Input: part model. Units: mm. Frame: model coordinates. Face numbers are marked on the shaded views. Give positions to 0.01 mm unless a question says otherwise; leave off trailing zeros. Loops run counter-clockwise (first coordinate to the right, second up) from the corner with the lowest first, then second, coordinate; pieces in that order, holes last. Notation, with made-up numbers: (45.25, 61.5) - (63.25, 61.5) arc R19 ccw to (63.25, 86.5) - close; hole circle Ø3 at (88, -32.5). An arc over 180 degrees is marked (long way). Answer as a JSON object with one key per item and string values. Group by question number.
(1) Section query D-D (y = 1.1). Return loops of the section in (x, z), plus the area to 3 significant figures.
(2) Mould query, pull axis X, two halves, no side actions, for the marked faces 1 and 2. Classes: +X half, -X half, draft (parallel to the pull), parting line (faces both ways), or undercut.
(3) Section query B-B (z = -68). Return loops of the section in (x, y), plus the area to 4 significant figures.
(4) Material intervals for L1, parallel to Z at x = 40.8, y = 0.2; L2, parallel to X at y = 0.3, z = -68; L3, parallel to Z at x = 28, y = 1.85, sorted ascending.
(5) Pin query (flat end, axial travel): P1, Ø3.5, axis at x = 40.8, z = -68, coming from the +Y side; P2, Ø0.8, axis at x = 19, y = 1.5, coming from the -Z side; P3, Ø0.8, axis at x = 21.5, y = 1.5, coming from the +Z side. Return the tip coordinate at first contact, or that it passes through.
(6) Section query A-A (x = 40.8). Return loops of the section in (y, z), plus the area to 3 significant figures.
(7) Section query C-C (z = -37). Return loops of the section in (x, y), plus the area to 3 significant figures.
Autodesk Fusion 360 part; units mm, degrees
sketch "Sketch1" plane through (0, 0, 0) normal (0, 1, 0) x (1, 0, 0)
  line L0 (0, 0) -> (43.3, 0)
  line L1 (43.3, 0) -> (43.3, 70.5)
  line L2 (43.3, 70.5) -> (0, 70.5)
  line L3 (0, 70.5) -> (0, 0)
  dimension "d1" = 43.3
  dimension "d2" = 70.5
extrude "Extrude1" add sketch "Sketch1" along normal blind 0.5
sketch "Sketch2" plane through (0, 0.5, 0) normal (0, 1, 0) x (-1, 0, 0)
  line L0 (0, -70.5) -> (0, 0)
  line L1 (0, 0) -> (-43.3, 0)
  line L2 (-43.3, 0) -> (-43.3, -70.5)
  line L3 (-43.3, -70.5) -> (0, -70.5) construction
  line L4 (-43.3, 0) -> (-43.3, -5) construction
  line L5 (-43.3, -70.5) -> (-43.3, -64.5) construction
  line L6 (-43.3, -64.5) -> (0, -64.5)
  line L7 (0, -64.5) -> (0, -6)
  line L8 (0, -6) -> (-43.3, -6)
  line L9 (-43.3, -6) -> (-43.3, -64.5)
  line L10 (0, -2.5) -> (-2.5, -2.5) construction
  line L11 (-43.3, -2.5) -> (-40.8, -2.5) construction
  circle A0 centre (-2.5, -68) radius 1.5
  circle A1 centre (-40.8, -68) radius 1.5
  circle A2 centre (-40.8, -2.5) radius 1.5
  circle A3 centre (-2.5, -2.5) radius 1.5
  dimension "d5" = 6
  dimension "d8" = 2.5
  dimension "d10" = 3
  dimension "d11" = 3
  dimension "d12" = 3
  dimension "d13" = 3
  dimension "d16" = 2.5
  dimension "d17" = 2.5
  dimension "d18" = 2.5
  dimension "d19" = 2.5
  dimension "d20" = 2.5
  dimension "d21" = 2.5
  dimension "d22" = 2.5
extrude "Extrude2" add sketch "Sketch2" along normal blind 1.67 contours L0 L2 L6 L7 L8 L9
extrude "Extrude3" cut sketch "Sketch2" against normal blind 5.737 contours A0 | A1 | A2 | A3
sketch "Sketch3" plane through (0, 2.17, 0) normal (0, 1, 0) x (-1, 0, 0)
  line L0 (-43.3, -6) -> (-43.3, -64.5)
  line L1 (-43.3, -64.5) -> (0, -64.5)
  line L2 (0, -64.5) -> (0, -6)
  line L3 (0, -6) -> (-43.3, -6)
  line L4 (-3.29, -9.29) -> (-40.01, -9.29)
  line L5 (-40.01, -9.29) -> (-40.01, -58.25)
  line L6 (-40.01, -58.25) -> (-3.29, -58.25)
  line L7 (-3.29, -58.25) -> (-3.29, -9.29)
  dimension "d23" = 36.72
  dimension "d24" = 48.96
  dimension "d25" = 3.29
  dimension "d26" = 3.29
extrude "Extrude4" cut sketch "Sketch3" against normal blind 0.5 contours L4 L5 L6 L7
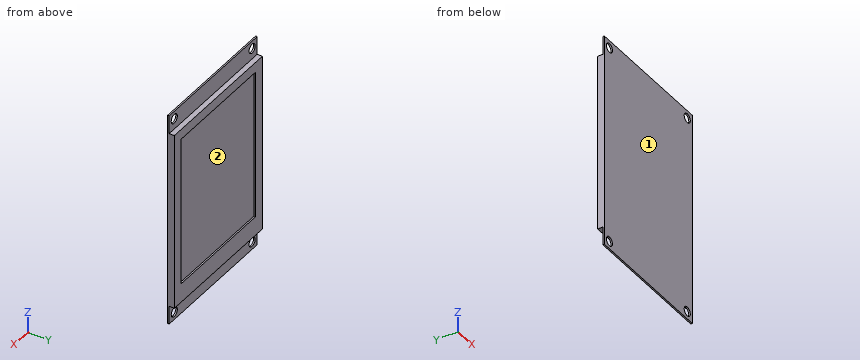
Recorded:
{
 "1": {"outline": "(0, -64.5) - (43.3, -64.5) - (43.3, -6) - (0, -6) - close", "area": "2,530 mm^2"},
 "2": {"face 1": "draft", "face 2": "undercut"},
 "3": {"outline": "(0, 0) - (1, 0) - (1, 0.5) - (0, 0.5) - close; (4, 0) - (39.3, 0) - (39.3, 0.5) - (4, 0.5) - close; (42.3, 0) - (43.3, 0) - (43.3, 0.5) - (42.3, 0.5) - close", "area": "18.65 mm^2"},
 "4": {"L1": "z = -70.5 to -69.5, -66.5 to -4, -1 to 0", "L2": "x = 0 to 1, 4 to 39.3, 42.3 to 43.3", "L3": "z = -64.5 to -58.25, -9.29 to -6"},
 "5": {"P1": "stops at y = 0.5", "P2": "stops at z = -64.5", "P3": "stops at z = -6"},
 "6": {"outline": "(0, -70.5) - (0.5, -70.5) - (0.5, -69.5) - (0, -69.5) - close; (0, -66.5) - (0.5, -66.5) - (0.5, -64.5) - (2.17, -64.5) - (2.17, -6) - (0.5, -6) - (0.5, -4) - (0, -4) - close; (0, -1) - (0.5, -1) - (0.5, 0) - (0, 0) - close", "area": "130 mm^2"},
 "7": {"outline": "(0, 0) - (43.3, 0) - (43.3, 2.17) - (40.01, 2.17) - (40.01, 1.67) - (3.29, 1.67) - (3.29, 2.17) - (0, 2.17) - close", "area": "75.6 mm^2"}
}
